Autodesk Inventor part; units mm, degrees
ref_plane "YZ Plane" through (0, 0, 0) normal (1, 0, 0) x (0, 1, 0)
ref_plane "XZ Plane" through (0, 0, 0) normal (0, 1, 0) x (-1, 0, 0)
ref_plane "XY Plane" through (0, 0, 0) normal (0, 0, 1) x (1, 0, 0)
sketch "Sketch1" plane through (0, 0, 0) normal (1, 0, 0) x (0, 1, 0)
  line L0 (0, 25.5) -> (0, -25.5)
  line L1 (0, 25.5) -> (8.33, 25.5)
  line L2 (0, -25.5) -> (8.33, -25.5)
  arc A0 (8.33, -25.5) -> (8.33, 25.5) centre (-164.8022, 0) ccw
  point P0 (0, 0)
  dimension "d0" = 51
  dimension "d1" = 8.33
  dimension "d2" = 8.33
  dimension "d3" = 175
revolve "Revolution1" add sketch "Sketch1" angle 360 about axis through (0, 0, 25.5) along (0, 0, -1)
sketch "Sketch2" plane through (0, 0, 25.5) normal (0, 0, 1) x (1, 0, 0)
  circle A0 centre (0, 0) radius 6
  dimension "d5" = 12
extrude "Extrusion1" cut sketch "Sketch2" against normal blind 2
sketch "Sketch3" plane through (0, 0, 23.5) normal (0, 0, 1) x (1, 0, 0)
  circle A0 centre (0, 0) radius 4
  dimension "d8" = 8
extrude "Extrusion2" cut sketch "Sketch3" against normal blind 2
fillet "Fillet1" radius 2.5 1 edges at (0, -8.33, 25.5)
mirror "Mirror1" about plane through (0, 0, 0) normal (0, 0, 1) of "Extrusion1", "Extrusion2", "Fillet1"
sketch "Sketch4" plane through (0, 0, 0) normal (0, 0, 1) x (1, 0, 0)
  circle A0 centre (0, 0) radius 4
  circle A1 centre (0, 0) radius 2
  point P0 (0, 0)
  dimension "d12" = 4
extrude "Extrusion3" cut sketch "Sketch4" along normal mid plane 805.5 contours A1
sketch "Sketch5" plane through (0, 0, 0) normal (1, 0, 0) x (0, 1, 0)
  line L0 (-0.25, -20) -> (0.25, -20)
  line L1 (0.25, -20) -> (0.25, 20)
  line L2 (0.25, 20) -> (-0.25, 20)
  line L3 (-0.25, 20) -> (-0.25, -20)
  line L4 (-0.25, -20) -> (0.25, 20) construction
  line L5 (0.25, -20) -> (-0.25, 20) construction
  point P0 (0, 0)
  dimension "d17" = 0.5
  dimension "d18" = 40
extrude "Extrusion4" cut sketch "Sketch5" along normal mid plane 40
properties part number "roller" material "Rubber"
Read the model definition and answer for the solid it produces. Units are mm, in the model's axes. A direction names the side the tool comes from. Give positions to 0.01 mm unless a question says otherwise; leave off trailing zeros. One line per item, written item: value. Start each with the question number.
(1) Find the intervals of material crossed by line 1 (Z direction, x = 3.5, y = 0); line 2 (Y direction, x = 5.25, z = 11); line 3 (Z direction, x = 2.25, y = 1.25), in increasing order.
(2) Flat-ended cylindrical pins translate along their axes: pin 1 Ø9 at (x, y) = (0, 0) entering from +Z; pin 2 Ø7 at (x, y) = (0, 0) entering from +Z; pin 3 Ø2.5 at (x, z) = (-4.5, -9.5) entering from -Y; pin 4 Ø2.5 at (x, y) = (0, 0) entering from -Z. Find the tip coordinate at first contact, or state that the pin passes through.
(3) A tool of negligible diameter and unlimited length cuts with its end or side. For faces 1 (the flat face through (2, -1, -21.5)), 2 (the flat face through (-1.42, -3.92, 23.5)), 3 (the flat face through (-6, -0.25, 0)), 4 (the cylindrical face through (1.847, -0.766, 0.301)), from which of +Z, -Z, +X, -X, +Y, -Y can it reach the whole face along a straight path? Write none if from no direction.
(4) Determine the mould class of faces 5 (the flat face through (1.42, -3.92, -23.5)), 6 (the flat face through (6, 0.25, 0)) for opening direction X: pulls with the +X half, pulls with the -X half, needs draft (parallel to the pull), parting line crosses it, or undercut.
Results below:
1. line 1: z = -21.5 to -20, 20 to 21.5
1. line 2: y = -8.34 to -0.25, 0.25 to 8.34
1. line 3: z = -21.5 to 21.5
2. pin 1: stops at z = 23.5
2. pin 2: stops at z = 21.5
2. pin 3: stops at y = -9.4
2. pin 4: passes through
3. face 1: -Z
3. face 2: +Z
3. face 3: +X, -X
3. face 4: +Z, -Z
4. face 5: undercut
4. face 6: needs draft
